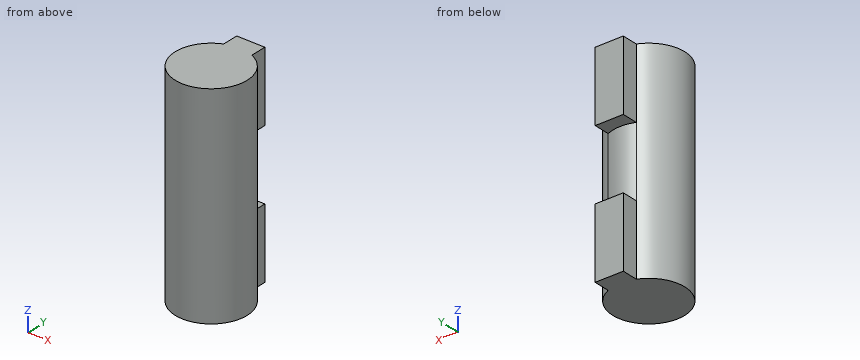
```python
from build123d import *

# Parameters (mm, degrees)
BOSS_EXTRUDE1_DEPTH = 30
CUT_EXTRUDE1_START  = -20
SKETCH2_R           = 7.822470446
SKETCH2_R_2         = 5.115
CUT_EXTRUDE1_DEPTH  = 10


with BuildPart() as part:
    # Sketch1 → Boss-Extrude1 (new body)
    with BuildSketch(Plane.XY):
        with BuildLine():
            Line((-2, 4.707783449), (-2, 7))
            Line((-2, 7), (2, 7))
            Line((2, 7), (2, 4.707783449))
            ThreePointArc((2, 4.707783449), (0, -5.115), (-2, 4.707783449))
        make_face()
    extrude(amount=BOSS_EXTRUDE1_DEPTH)

    # Sketch2 → Cut-Extrude1 (cut)
    with BuildSketch(Plane.XY.offset(30).offset(CUT_EXTRUDE1_START)):
        Circle(SKETCH2_R)
        with Locations(Location((0, 0, 0), (0, 0, 113.017162604))):
            Circle(SKETCH2_R_2, mode=Mode.SUBTRACT)
    extrude(amount=CUT_EXTRUDE1_DEPTH, mode=Mode.SUBTRACT)


solid = part.part
```
Could you check a few things on this model? Use its own coordinates, in mm. Round coordinates to 2 decimals unless told otherwise and drop trailing zeros. Loops run counter-clockwise (first coordinate to the right, second up) from the corner with the lowest first, then second, coordinate; pieces in that order, holes last.
Q1. Please list where these lines run through material, in increasing order: L1, parallel to Y at x = -0.25, z = 14.75; L2, parallel to X at y = 5.75, z = 4.5; L3, parallel to X at y = 3.25, z = 5.25.
Q2. I want a section at C-C (z = 15.5). Write out the boundary of the cut face in (x, y) (3 decimals), and give its area (3 significant figures).
Q3. I want a section at D-D (y = 2). Write out the boundary of the cut face in (x, z), and give its area (3 significant figures).
Q4. I want a section at B-B (x = 0). Write out the boundary of the cut face in (y, z) (3 decimals), and give its area (3 significant figures).
Q5. I want a section at A-A (y = 6.25). Write out the boundary of the cut face in (x, z).
Q6. For P1, Ø5, axis at x = 2.5, y = -3, coming from the -Z side; P2, Ø1.1, axis at y = 6, z = 7, coming from the +X side; P3, Ø1.8, axis at y = 6, z = 7, coming from the -X side; P4, Ø2.5, axis at y = 5.5, z = 24.5, coming from the +X side, each with a flat end and sliding along its axis, tell me the tip position at first contact or that it passes through.
Answer below:
1. L1: y = -5.11 to 5.11
1. L2: x = -2 to 2
1. L3: x = -3.95 to 3.95
2. outline: circle Ø10.23 at (0, 0)
2. area: 82.2 mm2
3. outline: (-4.71, 0) - (4.71, 0) - (4.71, 30) - (-4.71, 30) - close
3. area: 282 mm2
4. outline: (-5.115, 0) - (7, 0) - (7, 10) - (5.115, 10) - (5.115, 20) - (7, 20) - (7, 30) - (-5.115, 30) - close
4. area: 345 mm2
5. outline: (-2, 0) - (2, 0) - (2, 10) - (-2, 10) - close; (-2, 20) - (2, 20) - (2, 30) - (-2, 30) - close
6. P1: stops at z = 0
6. P2: stops at x = 2
6. P3: stops at x = -2
6. P4: stops at x = 2.85
